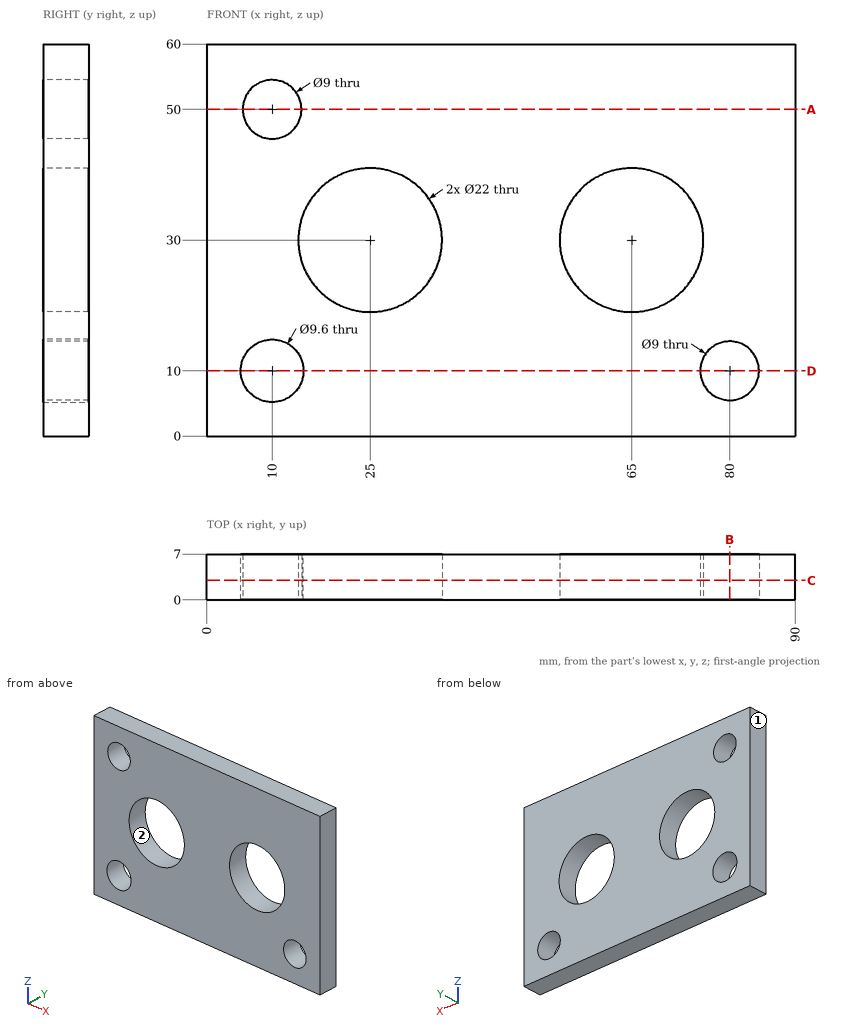
Verification items for this drawing (mm, ordinates from the low corner). Coordinates: 2 decimals unless noted, no trailing zeros. Order: outer loops, then holes, each group sorted by start corner. A loop starts at its lowest first (then second) coordinate and runs counter-clockwise, first axis right, second up. Notation, with made-up numbers: (79, 34.5) -> (123, 34.5) arc R16 ccw to (123, 57.5) -> close; hole circle Ø1 at (78, 10). An arc over 180 degrees is marked (long way). Answer as CSV lines item,"result". Start each with the question number.
1) Cross-section at A-A, the plane z = 50. Record the boundary of the cut face in (x, y), then the cut area to 3 significant figures.
2) Release check for a two-part mould opening along Z. For the marked faces 1 and 2 record: released by +Z, released by -Z, zero draft, split by the parting line, or undercut.
3) Gauge pin test, flat ends, axial feed: pin 1 Ø1 at (x, z) = (63.5, 17.5) entering from -Y; pin 2 Ø3 at (x, z) = (57.5, 26) entering from -Y. Record the tip position at first contact, or that the pin passes through.
4) Cross-section at C-C, the plane y = 3. Record the boundary of the cut face in (x, z).
5) Cross-section at B-B, the plane x = 80. Record the boundary of the cut face in (y, z).
6) Cross-section at D-D, the plane z = 10. Record the boundary of the cut face in (x, y), then the cut area to 3 significant figures.
7) Material ranges on L1, parallel to Z at x = 25, y = 4.25; L2, parallel to Z at x = 11, y = 2; L3, parallel to X at y = 3.75, z = 9, recorded low to high. Write a range as [from, to].
Conclusion:
1,outline,"(0, 0) -> (5.5, 0) -> (5.5, 7) -> (0, 7) -> close; (14.5, 0) -> (90, 0) -> (90, 7) -> (14.5, 7) -> close"
1,area,"567 mm²"
2,face 1,"zero draft"
2,face 2,"undercut"
3,pin 1,"stops at y = 0"
3,pin 2,"passes through"
4,outline,"(0, 0) -> (90, 0) -> (90, 60) -> (0, 60) -> close; hole circle Ø9.6 at (10, 10); hole circle Ø9 at (10, 50); hole circle Ø22 at (25, 30); hole circle Ø22 at (65, 30); hole circle Ø9 at (80, 10)"
5,outline,"(0, 0) -> (7, 0) -> (7, 5.5) -> (0, 5.5) -> close; (0, 14.5) -> (7, 14.5) -> (7, 60) -> (0, 60) -> close"
6,outline,"(0, 0) -> (5.2, 0) -> (5.2, 7) -> (0, 7) -> close; (14.8, 0) -> (75.5, 0) -> (75.5, 7) -> (14.8, 7) -> close; (84.5, 0) -> (90, 0) -> (90, 7) -> (84.5, 7) -> close"
6,area,"500 mm²"
7,L1,"z = [0, 19], [41, 60]"
7,L2,"z = [0, 5.31], [14.69, 45.61], [54.39, 60]"
7,L3,"x = [0, 5.31], [14.69, 75.61], [84.39, 90]"
